from build123d import *

# Parameters (mm, degrees)
BOSS_EXTRUDE2_DEPTH = 3
SKETCH1_8_R         = 1.5
BOSS_EXTRUDE5_DEPTH = 3
FILLET1_R           = 2
CUT_EXTRUDE1_REACH  = 5


with BuildPart() as part:
    # Sketch1 → Boss-Extrude2 (new body)
    with BuildSketch(Plane.XY):
        with BuildLine():
            Line((-19.985447982, 0.762803358), (-59.956343946, 2.288410074))
            ThreePointArc((-59.956343946, 2.288410074), (-55.730717245, 22.228071336), (-45.073672701, 39.602576043))
            Line((-45.073672701, 39.602576043), (-13.592462366, 14.67122922))
            ThreePointArc((-13.592462366, 14.67122922), (-18.172234131, 8.352838241), (-19.985447982, 0.762803358))
        make_face()
    extrude(amount=BOSS_EXTRUDE2_DEPTH)

    # Sketch1_8 → Boss-Extrude5 (add)
    with BuildSketch(Plane.XY):
        with BuildLine():
            Line((-7.103763171, 7.667553899), (-13.592462366, 14.67122922))
            ThreePointArc((-13.592462366, 14.67122922), (-18.172234131, 8.352838241), (-19.985447982, 0.762803358))
            Line((-19.985447982, 0.762803358), (-10.444898468, 0.398660247))
            Line((-10.444898468, 0.398660247), (14.68444307, -11.152001243))
            Line((14.68444307, -11.152001243), (18.025578366, -3.883107591))
            Line((18.025578366, -3.883107591), (-7.103763171, 7.667553899))
        make_face()
        Circle(SKETCH1_8_R, mode=Mode.SUBTRACT)
    extrude(amount=BOSS_EXTRUDE5_DEPTH)

    # Fillet1
    fillet1_edges = [part.edges().sort_by_distance(p)[0] for p in [
        (14.68444307, -11.152001243, 1.5),
        (18.025578366, -3.883107591, 1.5),
    ]]
    fillet(fillet1_edges, radius=FILLET1_R)

    # Sketch2 → Cut-Extrude1 (cut, up to next)
    with BuildSketch(Plane.XY.offset(3), mode=Mode.PRIVATE) as cut_extrude1_sk1:
        with BuildLine():
            Line((-52.047329922, 25.59444174), (-19.74209066, 9.708236522))
            ThreePointArc((-19.74209066, 9.708236522), (-20.223124653, 8.661710528), (-20.648728467, 7.591443388))
            Line((-20.648728467, 7.591443388), (-54.437556866, 20.013805296))
            ThreePointArc((-54.437556866, 20.013805296), (-53.315510448, 22.835418665), (-52.047329922, 25.59444174))
        make_face()
    cut_extrude1_tool1 = extrude(cut_extrude1_sk1.sketch, amount=-CUT_EXTRUDE1_REACH, mode=Mode.PRIVATE) & part.part
    add(cut_extrude1_tool1.solids().sort_by_distance((-39.233314, 16.803912, 3))[0], mode=Mode.SUBTRACT)
    # Sketch2 → Cut-Extrude1 (cut, up to next)
    with BuildSketch(Plane.XY.offset(3), mode=Mode.PRIVATE) as cut_extrude1_sk2:
        with BuildLine():
            Line((-56.231354546, 14.213893413), (-21.329134483, 5.391476812))
            ThreePointArc((-21.329134483, 5.391476812), (-21.58207174, 4.267807331), (-21.775854038, 3.132440087))
            Line((-21.775854038, 3.132440087), (-57.409069737, 8.25825114))
            ThreePointArc((-57.409069737, 8.25825114), (-56.898189132, 11.251492055), (-56.231354546, 14.213893413))
        make_face()
    cut_extrude1_tool2 = extrude(cut_extrude1_sk2.sketch, amount=-CUT_EXTRUDE1_REACH, mode=Mode.PRIVATE) & part.part
    add(cut_extrude1_tool2.solids().sort_by_distance((-41.869702, 8.279642, 3))[0], mode=Mode.SUBTRACT)
    # Sketch2 → Cut-Extrude1 (cut, up to next)
    with BuildSketch(Plane.XY.offset(3), mode=Mode.PRIVATE) as cut_extrude1_sk3:
        with BuildLine():
            Line((-49.08686154, 30.894660124), (-18.619154377, 11.718664185))
            ThreePointArc((-18.619154377, 11.718664185), (-17.980329977, 12.677055412), (-17.292222743, 13.600699711))
            Line((-17.292222743, 13.600699711), (-45.58858723, 35.856390146))
            ThreePointArc((-45.58858723, 35.856390146), (-47.402688122, 33.421327903), (-49.08686154, 30.894660124))
        make_face()
    cut_extrude1_tool3 = extrude(cut_extrude1_sk3.sketch, amount=-CUT_EXTRUDE1_REACH, mode=Mode.PRIVATE) & part.part
    add(cut_extrude1_tool3.solids().sort_by_distance((-34.882242, 24.593771, 3))[0], mode=Mode.SUBTRACT)


solid = part.part
Check sheet for the modelled part. Datum: model origin and axes. Units: mm. A direction names the side the tool comes from. Give positions to 0.01 mm unless a question says otherwise; leave off trailing zeros. Loops run counter-clockwise (first coordinate to the right, second up) from the corner with the lowest first, then second, coordinate; pieces in that order, holes last. Notation, with made-up numbers: M -27.5,40.5 L -2.5,40.5 A20 cw -2.5,61.5 Z; hole C 44.25,-25.75 d11. An arc over 180 degrees is marked long. Use a Markdown table: item, result. Add a question column.
Q1. Sectioned sample at D-D, the plane x = 0. Record the cut outline in (y, z), then the cut area to 3 significant figures.
Q2. Mould release check, pull along X, two halves, no side actions. Record for faces 3 (the cylindrical face through (14.417, -10.367, 1.521)), 4 (the cylindrical face through (-17.99, 12.66, 1.52)), 5 (the cylindrical face through (-56.906, 11.21, 1.521)), 6 (the flat face through (-10.3, 11.12, 1.48)): pulls with the +X half, pulls with the -X half, needs draft (parallel to the pull), parting line crosses it, or undercut.
Q3. Scan lines: line 1 along Y through (x, z) = (-40, 0.75); line 2 along X through (y, z) = (23, 0.5); line 3 along Y through (x, z) = (-37, 2.5). Record each from-to range of solid material in increasing order. Write a range as [from, to].
Q4. Tool access check on faces 1 (the flat face through (-39.34, 5.66, 1.52)), 2 (the flat face through (-29.55, 27.31, 1.48)). Record the directions out of +Z, -Z, +X, -X, +Y, -Y that give a thin tool (end or side, any length) a straight path to the whole face; none if there is none.
Q5. Go/stop test with flat-tipped pins: pin 1 (1.5 mm diameter, centred on x = -10, z = 1, fed in from +Y); pin 2 (12 mm diameter, centred on x = -27.5, y = 11.5, fed in from +Z); pin 3 (1 mm diameter, centred on y = 12.5, z = 2.5, fed in from +X). Record where each tip stops, or that it passes through.
Q6. Sectioned sample at C-C, the plane y = 27. Record the cut outline in (x, z).
Q7. Sectioned sample at B-B, the plane x = -24. Record the cut outline in (y, z).
Q8. Sectioned sample at A-A, the plane z = 2.25. Record the cut outline in (x, y).
Verdict:
| question | item | result |
|---|---|---|
| 1 | outline | M -4.4,0 L -1.5,0 L -1.5,3 L -4.4,3 Z; M 1.5,0 L 4.4,0 L 4.4,3 L 1.5,3 Z |
| 1 | area | 17.4 mm^2 |
| 2 | face 3 | parting line crosses it |
| 2 | face 4 | undercut |
| 2 | face 5 | undercut |
| 2 | face 6 | pulls with the +X half |
| 3 | line 1 | [1.53, 5.75], [10.11, 14.71], [19.67, 25.18], [31.46, 35.58] |
| 3 | line 2 | [-55.42, -53.24], [-46.77, -36.54], [-29.24, -24.11] |
| 3 | line 3 | [1.41, 5.32], [9.35, 13.6], [18.19, 23.29], [29.1, 33.21] |
| 4 | face 1 | +Z, -Z |
| 4 | face 2 | +Z, -Z, +X, +Y |
| 5 | pin 1 | y = 11.6 |
| 5 | pin 2 | z = 3 |
| 5 | pin 3 | x = -11.12 |
| 6 | outline | M -53.58,0 L -42.9,0 L -42.9,3 L -53.58,3 Z; M -34.33,0 L -29.16,0 L -29.16,3 L -34.33,3 Z |
| 7 | outline | M 0.92,0 L 3.45,0 L 3.45,3 L 0.92,3 Z; M 6.07,0 L 8.82,0 L 8.82,3 L 6.07,3 Z; M 11.8,0 L 15.11,0 L 15.11,3 L 11.8,3 Z; M 18.88,0 L 22.91,0 L 22.91,3 L 18.88,3 Z |
| 8 | outline | M -59.96,2.29 L -10.44,0.4 L 12.87,-10.32 A2 ccw 15.52,-9.33 L 17.19,-5.7 A2 ccw 16.21,-3.05 L -7.1,7.67 L -13.59,14.67 L -45.07,39.6 A60 ccw Z; hole M -57.41,8.26 L -21.78,3.13 A22 cw -21.33,5.39 L -56.23,14.21 A58 ccw Z; hole M -54.44,20.01 L -20.65,7.59 A22 cw -19.74,9.71 L -52.05,25.59 A58 ccw Z; hole M -49.09,30.89 L -18.62,11.72 A22 cw -17.29,13.6 L -45.59,35.86 A58 ccw Z; hole C 0,0 d3 |
